```python
from build123d import *

# Parameters (mm, degrees)
F1_DEPTH = 28.5
F2_DEPTH = 25
F3_DEPTH = 25
F4_DEPTH = 26
F5_DEPTH = 27.3


with BuildPart() as f1:
    # F0 (on Top) → F1 (new body)
    with BuildSketch(Plane.XY):
        Polygon((-29.307868, 0), (-20.729955, -10.960666), (-8.577912, -9.769289), (-7.784336, -9.462098), (-8.376737, -3.419617), (-10.007564, 1.667927), (-15.249622, 4.527232), align=None)
        Polygon((-8.577912, -9.769289), (-20.729955, -10.960666), (-16.250395, -14.699083), (-11.770834, -18.437501), (-7.529469, -12.061744), (-7.784336, -9.462098), align=None)
    extrude(amount=F1_DEPTH)

    # F0 (on Top) → F2 (join)
    with BuildSketch(Plane.XY):
        Polygon((-32.881998, -12.152042), (-57.186086, -5.718608), (-53.437501, -10.104167), (-46.770833, -12.1875), (-38.645834, -15.249623), (-28.437063, -15.249623), (-22.821563, -14.699083), (-16.250395, -14.699083), (-20.729955, -10.960666), align=None)
    extrude(amount=F2_DEPTH)

    # F0 (on Top) → F3 (join)
    with BuildSketch(Plane.XY):
        Polygon((6.19516, -4.050681), (-7.784336, -9.462098), (-7.529469, -12.061744), (0, -10.520834), (1.51446, -9.679468), (21.145836, -3.645833), (40.520836, 1.979167), (48.395412, 7.15981), (66.369534, 26.979169), (68.892609, 32.971472), (65.744534, 29.97532), (59.47917, 22.684125), (51.297057, 13.662031), (37.635021, 5.413258), (18.229166, 0), align=None)
    extrude(amount=F3_DEPTH)

    # F0 (on Top) → F4 (join)
    with BuildSketch(Plane.XY):
        with BuildLine():
            Line((-4.828904, 29.004751), (-9.769289, 33.835098))
            ThreePointArc((-9.769289, 33.835098), (-29.975189, 42.690738), (-50.990924, 35.97958))
            Line((-50.990924, 35.97958), (-57.900909, 30.260969))
            Line((-57.900909, 30.260969), (-62.428143, 19.776853))
            Line((-62.428143, 19.776853), (-62.904693, 6.671709))
            Line((-62.904693, 6.671709), (-57.186086, -5.718608))
            Line((-57.186086, -5.718608), (-32.881998, -12.152042))
            Line((-32.881998, -12.152042), (-20.729955, -10.960666))
            Line((-20.729955, -10.960666), (-29.307868, 0))
            Line((-29.307868, 0), (-15.249622, 4.527232))
            Line((-15.249622, 4.527232), (-10.007564, 1.667927))
            Line((-10.007564, 1.667927), (-8.376737, -3.419617))
            Line((-8.376737, -3.419617), (-7.784336, -9.462098))
            Line((-7.784336, -9.462098), (6.19516, -4.050681))
            Line((6.19516, -4.050681), (18.229166, 0))
            Line((18.229166, 0), (37.635021, 5.413258))
            Line((37.635021, 5.413258), (51.297057, 13.662031))
            Line((51.297057, 13.662031), (59.47917, 22.684125))
            Line((59.47917, 22.684125), (65.744534, 29.97532))
            Line((65.744534, 29.97532), (68.892609, 32.971472))
            Line((68.892609, 32.971472), (71.14584, 42.604171))
            Line((71.14584, 42.604171), (71.14584, 46.145838))
            Line((71.14584, 46.145838), (64.895838, 46.145838))
            Line((64.895838, 46.145838), (59.270833, 43.020837))
            Line((59.270833, 43.020837), (55.186109, 34.90815))
            Line((55.186109, 34.90815), (51.770836, 43.4375))
            Line((51.770836, 43.4375), (44.479169, 46.145838))
            Line((44.479169, 46.145838), (37.635021, 46.145838))
            Line((37.635021, 46.145838), (37.635021, 42.274959))
            Line((37.635021, 42.274959), (39.190768, 34.62882))
            Line((39.190768, 34.62882), (42.812504, 28.854169))
            Line((42.812504, 28.854169), (43.496898, 25.49053))
            Line((43.496898, 25.49053), (37.8928, 19.333061))
            Line((37.8928, 19.333061), (31.963997, 16.239772))
            Line((31.963997, 16.239772), (19.062029, 15.964448))
            Line((19.062029, 15.964448), (5.480333, 21.683058))
            Line((5.480333, 21.683058), (-4.828904, 29.004751))
        make_face()
        with BuildLine():
            ThreePointArc((-33.213809, 16.979167), (-28.598407, 17.594186), (-26.130475, 13.645833))
            Line((-26.130475, 13.645833), (-28.42214, 11.562501))
            Line((-28.42214, 11.562501), (-30.428787, 13.704629))
            Line((-30.428787, 13.704629), (-33.213809, 15.102518))
            Line((-33.213809, 15.102518), (-35.420312, 15.102518))
            Line((-35.420312, 15.102518), (-33.213809, 16.979167))
        make_face(mode=Mode.SUBTRACT)
    extrude(amount=F4_DEPTH)

    # F0 (on Top) → F5 (join)
    with BuildSketch(Plane.XY):
        with BuildLine():
            Line((-28.42214, 11.562501), (-26.130475, 13.645833))
            ThreePointArc((-26.130475, 13.645833), (-28.598407, 17.594186), (-33.213809, 16.979167))
            Line((-33.213809, 16.979167), (-35.420312, 15.102518))
            Line((-35.420312, 15.102518), (-33.213809, 15.102518))
            Line((-33.213809, 15.102518), (-30.428787, 13.704629))
            Line((-30.428787, 13.704629), (-28.42214, 11.562501))
        make_face()
    extrude(amount=F5_DEPTH)


solid = f1.part
```
Geometry: final body of the model. Coordinates: model frame, mm. A direction names the side the tool comes from. Coordinates: 2 decimals unless noted, no trailing zeros. Order: outer loops, then holes, each group sorted by start corner. A loop starts at its lowest first (then second) coordinate and runs counter-clockwise, first axis right, second up. Notation, with made-up numbers: M 67,-35.75 L 83,-35.75 A19 ccw 83,-8.75 Z; hole C 81,31 d9. An arc over 180 degrees is marked long. Answer as CSV lines item,"result".
Q1. Set-up query: faces 4 (the flat face through (-12.592, 3.078, 27.232)), 5 (the flat face through (-25.08, -5.4, 27.23)), 6 (the flat face through (53.502, 39.113, 12.818)), 7 (the flat face through (-34, -15.25, 12)). Return all of +Z, -Z, +X, -X, +Y, -Y with unobstructed straight access to the full face (end or side cutting, diameter ignored); none if empty.
Answers:
face 4,"+Z, +X, +Y"
face 5,"+Z, -X, -Y"
face 6,"+Z, -Z, +Y"
face 7,"+Z, -Z, -X, -Y"
Q2. First-contact query: P1, Ø17.5, axis at x = 22, y = 20.5, coming from the +Z side; P2, Ø2, axis at x = -20.5, z = 17.5, coming from the -Y side; P3, Ø1.2, axis at y = 44.5, z = 10, coming from the -X side (3 decimals). Flat tips, straight axial feed; report the tip coordinate or a pass-through.
Answers:
P1,"stops at z = 26"
P2,"stops at y = -14.7"
P3,"stops at x = 37.635"
Q3. Section C-C on y = 9. Return the cut outline in (x, z).
Answers:
outline,"M -62.82,0 L 50.06,0 L 50.06,25 L 43.58,25 L 43.58,26 L -62.82,26 Z"
Q4. Section B-B on x = -13. Return the cut outline in (y, z).
Answers:
outline,"M -17.41,0 L 36.59,0 L 36.59,26 L 3.3,26 L 3.3,28.5 L -17.41,28.5 Z"
Q5. Section A-A on y = 40.5. Return the cut outline in (x, z).
Answers:
outline,"M -43.19,0 L -20,0 L -20,26 L -43.19,26 Z; M 38,0 L 52.95,0 L 52.95,26 L 38,26 Z; M 58,0 L 70.65,0 L 70.65,26 L 58,26 Z"
Q6. Draft query along X for faces 1 (the flat face through (67.6, 29.9, 12.3)), 2 (the flat face through (-22.18, 2.295, 27.232)), 3 (the flat face through (-25.67, -14.98, 12.32)). Return one class per face: pulls with the +X half, pulls with the -X half, needs draft (parallel to the pull), parting line crosses it, or undercut.
Answers:
face 1,"pulls with the +X half"
face 2,"pulls with the -X half"
face 3,"undercut"
Q7. Line query: probe 1 along X at (y, z) = (21, 6); probe 2 along Z at (x, y) = (46.5, 29.5); probe 3 along X at (y, z) = (31, 10.5). Output: solid intervals per line, ascending. Write a range as [from, to].
Answers:
probe 1,"x = [-61.9, 7.1], [39.41, 60.95]"
probe 2,"z = [0, 26]"
probe 3,"x = [-57.01, -6.87], [41.47, 68.06]"
